Could you check a few things on this model? Use its own coordinates, in mm. A direction names the side the tool comes from. Coordinates: 2 decimals unless noted, no trailing zeros. Order: outer loops, then holes, each group sorted by start corner. A loop starts at its lowest first (then second) coordinate and runs counter-clockwise, first axis right, second up. Notation, with made-up numbers: M 35.5,-38.75 L 81.5,-38.75 A18 cw 81.5,-32.75 Z; hole C 0.5,4.5 d7. An arc over 180 degrees is marked long. Put each result on its own line as item: value. Start each with the question number.
```python
from build123d import *

# Parameters (mm, degrees)
EXTRUDE_1_DEPTH = 700


with BuildPart() as part:
    # Эскиз1 → Бобышка-Вытянуть1 (new body)
    with BuildSketch(Plane.XY):
        with BuildLine():
            Line((-25.388920969, 15), (-1.388920969, 15))
            ThreePointArc((-1.388920969, 15), (0.732399375, 14.121320344), (1.611079031, 12))
            Line((1.611079031, 12), (1.611079031, -12))
            ThreePointArc((1.611079031, -12), (0.732399375, -14.121320344), (-1.388920969, -15))
            Line((-1.388920969, -15), (-25.388920969, -15))
            ThreePointArc((-25.388920969, -15), (-27.510241313, -14.121320344), (-28.388920969, -12))
            Line((-28.388920969, -12), (-28.388920969, 12))
            ThreePointArc((-28.388920969, 12), (-27.510241313, 14.121320344), (-25.388920969, 15))
        make_face()
        with BuildLine():
            Line((-24.388920969, 13), (-2.388920969, 13))
            ThreePointArc((-2.388920969, 13), (-0.974707407, 12.414213562), (-0.388920969, 11))
            Line((-0.388920969, 11), (-0.388920969, -11))
            ThreePointArc((-0.388920969, -11), (-0.974707407, -12.414213562), (-2.388920969, -13))
            Line((-2.388920969, -13), (-24.388920969, -13))
            ThreePointArc((-24.388920969, -13), (-25.803134531, -12.414213562), (-26.388920969, -11))
            Line((-26.388920969, -11), (-26.388920969, 11))
            ThreePointArc((-26.388920969, 11), (-25.803134531, 12.414213562), (-24.388920969, 13))
        make_face(mode=Mode.SUBTRACT)
    extrude(amount=EXTRUDE_1_DEPTH)

    # Зеркальное отражение1: part across plane


with BuildPart() as part_1:
    add(part.part)
    add(part.part.mirror(Plane(origin=(-25.388920969, -12, 0), x_dir=(1, 0, 0), z_dir=(0, 0, 1))))


solid = part_1.part
```
Item 1: If we section it at A-A on x = -10: Write out the boundary of the cut face in (y, z).
Item 2: If we section it at C-C on y = -4.5: Write out the boundary of the cut face in (x, z).
Item 3: If we mould it in two halves opening along X, with no side actions, what happens to faces 3 (the flat face through (-26.389, 0, 10)), 4 (the flat face through (-13, -13, 10)), 5 (the flat face through (0, 0, -700)), 6 (the flat face through (-28.389, 0, 10))? For each: released by +X, released by -X, zero draft, split by the parting line, or undercut.
Item 4: I need wall thicknesses on probe 1 along X at (y, z) = (2.75, 5); probe 2 along Y at (x, z) = (-16, -289.5); probe 3 along X at (y, z) = (-11.75, 312). Which ranges of each line are inside material? Lowest first, please.
Item 5: If we section it at B-B on z = -284.5: Write out the boundary of the cut face in (x, y).
Item 6: For faces 1 (the flat face through (1.611, 0, 10)), 2 (the flat face through (-0.389, 0, 10)), which set-ups out of +Z, -Z, +X, -X, +Y, -Y let a thin tool reach every point of the face, with its end or its side?
Geometry check:
1. outline: M -15,-700 L -13,-700 L -13,700 L -15,700 Z; M 13,-700 L 15,-700 L 15,700 L 13,700 Z
2. outline: M -28.39,-700 L -26.39,-700 L -26.39,700 L -28.39,700 Z; M -0.39,-700 L 1.61,-700 L 1.61,700 L -0.39,700 Z
3. face 3: undercut
3. face 4: undercut
3. face 5: zero draft
3. face 6: released by -X
4. probe 1: x = -28.39 to -26.39, -0.39 to 1.61
4. probe 2: y = -15 to -13, 13 to 15
4. probe 3: x = -28.39 to -26.24, -0.53 to 1.61
5. outline: M -28.39,-12 A3 ccw -25.39,-15 L -1.39,-15 A3 ccw 1.61,-12 L 1.61,12 A3 ccw -1.39,15 L -25.39,15 A3 ccw -28.39,12 Z; hole M -26.39,-11 A2 ccw -24.39,-13 L -2.39,-13 A2 ccw -0.39,-11 L -0.39,11 A2 ccw -2.39,13 L -24.39,13 A2 ccw -26.39,11 Z
6. face 1: +Z, -Z, +X, +Y, -Y
6. face 2: +Z, -Z
